Job drawing, mm, ordinate dimensions from the low corner. One solid piece. A direction names the side the tool comes from. Give positions to 0.01 mm unless a question says otherwise; leave off trailing zeros. Write each loop counter-clockwise with the first axis right and the second up, starting at its lowest first coordinate (ties: lowest second). Pieces come first, ordered by that corner, then holes. Notation, with made-up numbers: (-9, -29) - (13, -29) arc R30 ccw to (13, -4) - close; hole circle Ø5 at (-17, 4.5). An arc over 180 degrees is marked (long way). Answer in a Markdown table with one row per item. Add a question column.
1. Band-saw the part on C-C on z = 170. Write the cut outline in (x, y), plus the area to 3 significant figures.
2. Drop flat-ended pins along their axis: pin 1 Ø6.5 at (x, y) = (168.5, 8) entering from -Z; pin 2 Ø13 at (y, z) = (60.5, 3.5) entering from +X; pin 3 Ø9.5 at (y, z) = (30, 25.5) entering from -X; pin 4 Ø3.5 at (y, z) = (69.5, 7.5) entering from -X. Give the stop position or say it passes through.
3. Probe line 1 along Z through (x, y) = (264.5, 10.5); line 2 along Y through (x, z) = (418.4, 148); line 3 along X through (y, z) = (56, 233). List the from-to ranges inside material, lowest first.
4. Which spindle directions (+Z, -Z, +X, -X, +Y, -Y) get a long thin tool onto all of the face, cutting with end or side? Do the marked faces 1, 2 and 3. Say none if no direction does.
5. Band-saw the part on B-B on x = 114. Write the cut outline in (y, z), plus the area to 3 significant figures.
6. Band-saw the part on A-A on y = 68. Write the cut outline in (x, z), plus the area to 3 significant figures.
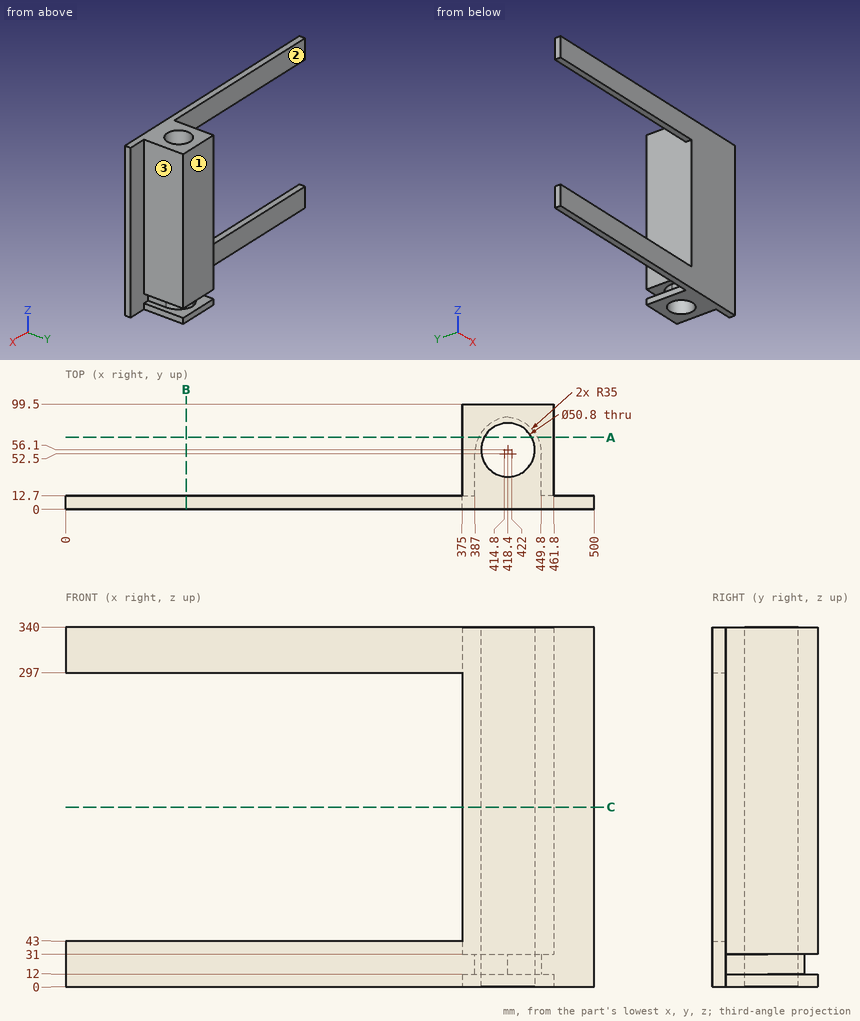
Values:
| question | item | result |
|---|---|---|
| 1 | outline | (375, 0) - (500, 0) - (500, 12.7) - (461.8, 12.7) - (461.8, 99.5) - (375, 99.5) - close; hole circle Ø50.8 at (418.4, 56.1) |
| 1 | area | 7,090 mm² |
| 2 | pin 1 | stops at z = 0 |
| 2 | pin 2 | stops at x = 461.8 |
| 2 | pin 3 | stops at x = 387 |
| 2 | pin 4 | stops at x = 375 |
| 3 | line 1 | z = 0 to 43, 297 to 340 |
| 3 | line 2 | y = 0 to 30.7, 81.5 to 99.5 |
| 3 | line 3 | x = 375 to 393, 443.8 to 461.8 |
| 4 | face 1 | +Z, -Z, +X, -X, +Y |
| 4 | face 2 | +Z, -Z, -X, +Y |
| 4 | face 3 | +Z, -Z, +X, +Y |
| 5 | outline | (0, 0) - (12.7, 0) - (12.7, 43) - (0, 43) - close; (0, 297) - (12.7, 297) - (12.7, 340) - (0, 340) - close |
| 5 | area | 1,090 mm² |
| 6 | outline | (375, 0) - (395.96, 0) - (395.96, 340) - (375, 340) - (375, 31) - (390.62, 31) - (390.62, 12) - (375, 12) - close; (440.84, 0) - (461.8, 0) - (461.8, 12) - (446.18, 12) - (446.18, 31) - (461.8, 31) - (461.8, 340) - (440.84, 340) - close |
| 6 | area | 13,700 mm² |
